Check sheet for the drawn part. Datum: minimum x, y, z corner. Units: mm. A direction names the side the tool comes from. Give positions to 0.01 mm unless a question says otherwise; leave off trailing zeros. Order: outer loops, then holes, each group sorted by start corner. A loop starts at its lowest first (then second) coordinate and runs counter-clockwise, first axis right, second up. Notation, with made-up numbers: (22, 49) -> (51, 49) arc R22 cw to (51, 55) -> close; hole circle Ø6 at (76, -11.75). An arc over 180 degrees is marked (long way). Return JSON: item names as keys, results as strings. Group by question number.
(1) Depth check by flat-ended pin: pin 1 Ø12 at (x, z) = (48, 7.5) entering from -Y; pin 2 Ø1 at (x, y) = (47.5, 92) entering from +Z (1 decimal); pin 3 Ø6 at (x, z) = (6, 19.5) entering from +Y. Enter the tip coordinate at first touch or a pass-through.
(2) Cross-section at B-B on y = 94. Enter the section's corners in (x, z).
(3) Cross-section at C-C on z = 15.75. Enter the section's corners in (x, y).
(4) Thickness scan on line 1 along Z through (x, y) = (44, 115.5); line 2 along Z through (x, y) = (53, 90); line 3 along Y through (x, z) = (9.5, 20.75). Record the ranges inside material, lowest first.
(5) Cross-section at A-A on x = 16. Enter the section's corners in (y, z) (1 decimal), then the cut area to 3 significant figures.
(6) Tool access check on the marked faces 1 and 2. Record the directions out of +Z, -Z, +X, -X, +Y, -Y that give a thin tool (end or side, any length) a straight path to the whole face; none if there is none.
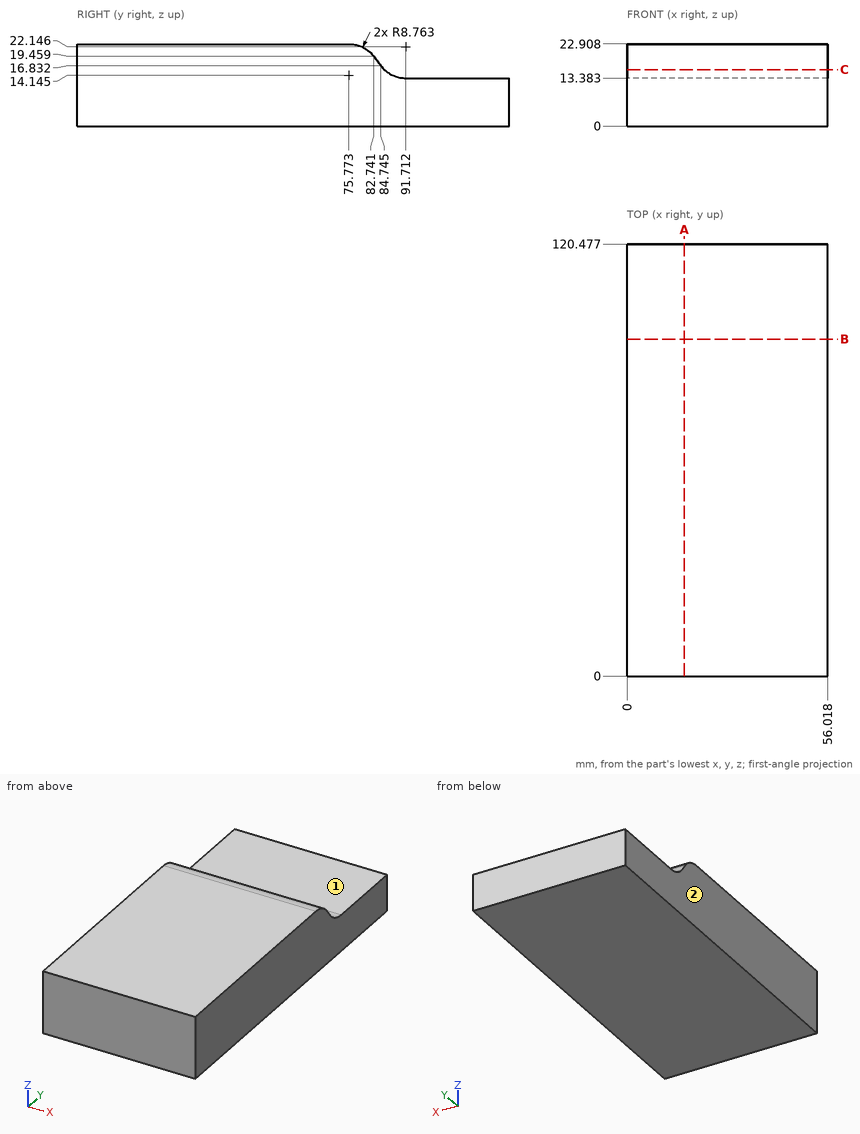
Verdict:
{
 "1": {"pin 1": "y = 0", "pin 2": "z = 13.4", "pin 3": "y = 85.01"},
 "2": {"outline": "(0, 0) -> (56.02, 0) -> (56.02, 13.38) -> (0, 13.38) -> close"},
 "3": {"outline": "(0, 0) -> (56.02, 0) -> (56.02, 85.72) -> (0, 85.72) -> close"},
 "4": {"line 1": "0 to 13.38", "line 2": "0 to 13.55", "line 3": "0 to 81.53"},
 "5": {"outline": "(0, 0) -> (120.5, 0) -> (120.5, 13.4) -> (91.7, 13.4) arc R8.8 cw to (84.7, 16.8) -> (82.7, 19.5) arc R8.8 ccw to (75.8, 22.9) -> (0, 22.9) -> close", "area": "2,410 mm²"},
 "6": {"face 1": "+Z, +X, -X, +Y", "face 2": "+Z, -Z, -X, +Y, -Y"}
}
